Work out the finished part from the listing and answer in its coordinate system (mm). A direction names the side the tool comes from. Coordinates: 2 decimals unless noted, no trailing zeros. Order: outer loops, then holes, each group sorted by start corner. A loop starts at its lowest first (then second) coordinate and runs counter-clockwise, first axis right, second up. Notation, with made-up numbers: M -5.75,-17 L 22.25,-17 A29 cw 22.25,7 Z; hole C 81,39.5 d2. An arc over 180 degrees is marked long. Use a Markdown table: item, result.
Autodesk Inventor part; units mm, degrees
ref_plane "YZ Plane" through (0, 0, 0) normal (1, 0, 0) x (0, 1, 0)
ref_plane "XZ Plane" through (0, 0, 0) normal (0, 1, 0) x (-1, 0, 0)
ref_plane "XY Plane" through (0, 0, 0) normal (0, 0, 1) x (1, 0, 0)
sketch "Main Sketch" plane through (0, 0, 0) normal (0, 1, 0) x (-1, 0, 0)
  line L0 (-57.375, -12.0472) -> (-57.375, 12.0472)
  line L1 (-57.375, 12.0472) -> (47.625, -10) construction
  line L2 (47.625, 10) -> (-57.375, -12.0472) construction
  circle A0 centre (47.625, 0) radius 7
  arc A1 (47.625, -10) -> (47.625, 10) centre (47.625, 0) ccw
  line L3 (-40.875, 17.5) -> (-57.375, 17.5)
  line L4 (-57.375, 17.5) -> (-57.375, -17.5)
  line L5 (-57.375, -17.5) -> (-40.875, -17.5)
  line L6 (-40.875, 17.5) -> (-57.375, -17.5) construction
  line L7 (-57.375, 17.5) -> (-40.875, -17.5) construction
  line L8 (47.625, -10) -> (-40.875, -10)
  line L9 (-40.875, -17.5) -> (-40.875, -10)
  line L10 (-40.875, 10) -> (-40.875, 17.5)
  line L11 (-40.875, 10) -> (47.625, 10)
  point P0 (0, 0)
  point P1 (-49.125, 0)
  dimension "d3" = 14
  dimension "d4" = 105
  dimension "d13" = 16.5
  dimension "d14" = 35
  dimension "d15" = 0
  dimension "d18" = 20
extrude "Main Extrusion" add sketch "Main Sketch" along normal blind 4
sketch "Screw Holes Sketch" plane through (0, 4, 0) normal (0, 1, 0) x (1, 0, 0)
  circle A0 centre (46.125, -8.75) radius 2
  line L0 (57.375, 17.5) -> (40.875, 17.5)
  line L1 (40.875, -17.5) -> (57.375, -17.5)
  line L2 (35.2664, 0) -> (65.7891, 0)
  line L3 (51.375, -27.0398) -> (51.375, 30.2346) construction
  line L4 (57.375, -17.5) -> (57.375, 17.5)
  line L5 (40.875, -10) -> (40.875, -17.5)
  circle A1 centre (46.125, 8.75) radius 2
  line L6 (51.375, 27.0398) -> (51.375, -30.2346) construction
  point P0 (0, 0)
  dimension "d21" = 4
  dimension "d22" = 35
  dimension "d23" = 6
  dimension "d24" = 5.25
  dimension "d25" = 5.25
  dimension "d26" = 10.5
  dimension "d27" = 8.75
  dimension "d28" = 17.5
extrude "Screw Holes Cut" cut sketch "Screw Holes Sketch" against normal through all
fillet "Smoooooooooooooooooth" radius 6 2 edges at (40.875, 2, -17.5) (40.875, 2, 17.5)
sketch "Side Axel Hole Sketch" plane through (-47.625, 0, 10) normal (0, 0, 1) x (1, 0, 0)
  line L0 (88.5, 4) -> (88.5, 0)
  line L1 (0, 0) -> (0, 4)
  line L2 (44.25, -12.0383) -> (44.25, 22.7681) construction
  line L3 (88.5, 0) -> (0, 0)
  line L4 (0, 4) -> (88.5, 4)
  circle A0 centre (44.25, 4) radius 1.5
  point P0 (47.625, 0)
  dimension "d32" = 88.5
  dimension "d33" = 44.25
  dimension "d34" = 44.25
  dimension "d35" = 4
  dimension "d41" = 3
extrude "Side Axel Hole Cut" cut sketch "Side Axel Hole Sketch" against normal blind 20 contours A0 L4 | L4 A0
sketch "Side Hole Extension Sketch" plane through (-47.625, 0, 10) normal (0, 0, 1) x (1, 0, 0)
  arc A0 (42.75, 4) -> (45.75, 4) centre (44.25, 4) ccw
  circle A1 centre (44.25, 4) radius 3
  circle A2 centre (44.25, 4) radius 1.5
  point P0 (47.625, 0)
  dimension "d44" = 6
extrude "Side Hole Extrusion" add sketch "Side Hole Extension Sketch" against normal blind 20
sketch "Body Holes Sketch" plane through (0, 4, 0) normal (0, 1, 0) x (1, 0, 0)
  line L0 (-37.625, 8) -> (-8.375, 8)
  line L1 (-8.375, 8) -> (-8.375, 4)
  line L2 (-8.375, 4) -> (-37.625, 4)
  line L3 (-37.625, 4) -> (-37.625, 8)
  line L4 (-6.375, -10) -> (-6.375, 10)
  circle A0 centre (-47.625, 0) radius 7
  line L5 (-47.625, 7) -> (-47.625, -13.5384) construction
  line L6 (-6.375, 10) -> (-47.625, 10)
  line L7 (-47.625, 1) -> (-47.625, -19.5384) construction
  line L8 (-37.625, 2) -> (-8.375, 2)
  line L9 (-8.375, 2) -> (-8.375, -2)
  line L10 (-8.375, -2) -> (-37.625, -2)
  line L11 (-37.625, -2) -> (-37.625, 2)
  line L12 (-47.625, -5) -> (-47.625, -25.5384) construction
  line L13 (-37.625, -4) -> (-8.375, -4)
  line L14 (-8.375, -4) -> (-8.375, -8)
  line L15 (-8.375, -8) -> (-37.625, -8)
  line L16 (-37.625, -8) -> (-37.625, -4)
  line L17 (1.625, 8) -> (39.625, 8)
  line L18 (39.625, 8) -> (39.625, 4)
  line L19 (39.625, 4) -> (1.625, 4)
  line L20 (1.625, 4) -> (1.625, 8)
  line L21 (-0.375, 10) -> (-0.375, -10)
  line L22 (40.875, 10) -> (-0.375, 10)
  line L23 (1.625, -2) -> (1.625, 2)
  line L24 (39.625, -2) -> (1.625, -2)
  line L25 (39.625, 2) -> (39.625, -2)
  line L26 (1.625, 2) -> (39.625, 2)
  line L27 (1.625, -8) -> (1.625, -4)
  line L28 (39.625, -8) -> (1.625, -8)
  line L29 (39.625, -4) -> (39.625, -8)
  line L30 (1.625, -4) -> (39.625, -4)
  point P0 (0, 0)
  dimension "d77" = 4
  dimension "d78" = 2
  dimension "d79" = 10
  dimension "d80" = 2
  dimension "d83" = 6
  dimension "d88" = 2
  dimension "d89" = 2
  dimension "d90" = 4
  dimension "d91" = 38
  dimension "d94" = 6
extrude "Swiss-ified" cut sketch "Body Holes Sketch" against normal through all contours L0 L1 L2 L3 | L8 L9 L10 L11 | L13 L14 L15 L16 | L17 L18 L19 L20 | L23 L26 L25 L24 | L27 L30 L29 L28
properties part number "Side V2.1"
1. Flat-ended cylindrical pins translate along their axes: P1, Ø3, axis at x = 10.5, y = 5, coming from the -Z side; P2, Ø1, axis at x = -4.5, z = 9, coming from the +Y side; P3, Ø2.5, axis at x = 46.125, z = 8.75, coming from the -Y side; P4, Ø1.2, axis at x = -17.5, y = 2.5, coming from the +Z side. Find the tip coordinate at first contact, or state that the pin passes through.
Answers below:
| item | result |
|---|---|
| P1 | z = -10 |
| P2 | y = 6.93 |
| P3 | through |
| P4 | z = 10 |
2. Find the intervals of material crossed by probe 1 along Z at (x, y) = (14.5, 3.5); probe 2 along X at (y, z) = (3.25, 9) (3 decimals); probe 3 along Y at (x, z) = (-14, 3), in increasing order.
Answers below:
| item | result |
|---|---|
| probe 1 | -10 to -8, -4 to -2, 2 to 4, 8 to 10 |
| probe 2 | -51.984 to -4.674, -2.076 to 44.141, 48.109 to 57.375 |
| probe 3 | 0 to 4 |
3. For faces 1 (the face through (-23, 2, 2)), 2 (the face through (42, 4, 0)), 3 (the face through (-4, 2, 10)), determine the directions among +Z, -Z, +X, -X, +Y, -Y from which every point of the face is accessible in a straight line to the end or side of a thin tool.
Answers below:
| item | result |
|---|---|
| face 1 | +Y, -Y |
| face 2 | +Z, -Z, +X, +Y |
| face 3 | +Z, -X, +Y, -Y |
4. Section D-D on z = -15 is taken. Determine the outline of the cut face in (x, y) (3 decimals).
Answers below:
| item | result |
|---|---|
| outline | M 42.002,0 L 57.375,0 L 57.375,4 L 42.002,4 Z |
5. Section B-B on x = -25.5 is taken. Determine the outline of the cut face in (y, z).
Answers below:
| item | result |
|---|---|
| outline | M 0,-10 L 4,-10 L 4,-8 L 0,-8 Z; M 0,-4 L 4,-4 L 4,-2 L 0,-2 Z; M 0,2 L 4,2 L 4,4 L 0,4 Z; M 0,8 L 4,8 L 4,10 L 0,10 Z |
6. Section C-C on z = -5 is taken. Determine the outline of the cut face in (x, y) (3 decimals), then the cut area to 3 significant figures.
Answers below:
| item | result |
|---|---|
| outline | M -56.285,0 L -52.524,0 L -52.524,4 L -56.285,4 Z; M -42.726,0 L -37.625,0 L -37.625,4 L -42.726,4 Z; M -8.375,0 L 1.625,0 L 1.625,4 L -0.375,4 A3 ccw -6.375,4 L -8.375,4 Z; M 39.625,0 L 57.375,0 L 57.375,4 L 39.625,4 Z; hole C -3.375,4 d3 |
| area | 154 mm² |
7. Section A-A on z = 0 is taken. Determine the outline of the cut face in (x, y) (3 decimals), then the cut area to 3 significant figures.
Answers below:
| item | result |
|---|---|
| outline | M -57.625,0 L -54.625,0 L -54.625,4 L -57.625,4 Z; M -40.625,0 L -37.625,0 L -37.625,4 L -40.625,4 Z; M -8.375,0 L 1.625,0 L 1.625,4 L -0.375,4 A3 ccw -6.375,4 L -8.375,4 Z; M 39.625,0 L 57.375,0 L 57.375,4 L 39.625,4 Z; hole C -3.375,4 d3 |
| area | 142 mm² |
8. For a pull along X with two mould halves and no side action, classify faces 4 (the face through (-37.625, 2, 0)), 5 (the face through (57.375, 2, 0)), 6 (the face through (-57.623, 1.972, 0.22)), 7 (the face through (52, 2, -17.5)) as +X half, -X half, draft (parallel to the pull), parting line (faces both ways), or undercut.
Answers below:
| item | result |
|---|---|
| face 4 | undercut |
| face 5 | +X half |
| face 6 | -X half |
| face 7 | draft |
